Autodesk Fusion 360 part; units mm, degrees
sketch "Sketch1" plane through (0, 0, 0) normal (0, 0, 1) x (1, 0, 0)
  line L0 (0, 0) -> (23, 0)
  line L1 (23, 0) -> (23, 19)
  line L2 (23, 19) -> (0, 19)
  line L3 (0, 19) -> (0, 0)
  line L4 (0, 0) -> (23, 19) construction
  line L5 (14, -5.5) -> (9, -5.5) construction
  line L6 (9, -5.5) -> (9, 24.5)
  line L7 (9, 24.5) -> (14, 24.5) construction
  line L8 (14, 24.5) -> (14, -5.5)
  line L9 (14, -5.5) -> (9, 24.5) construction
  line L10 (9, -5.5) -> (14, 24.5) construction
  line L11 (-3, 22) -> (-3, -3)
  line L12 (-3, -3) -> (26, -3)
  line L13 (26, -3) -> (26, 22)
  line L14 (26, 22) -> (-3, 22)
  point P0 (11.5, 9.5)
  dimension "d1" = 23
  dimension "d2" = 19
  dimension "d5" = 5
  dimension "d6" = 3
  dimension "d11" = 30
extrude "Extrude4" add sketch "Sketch1" along normal blind 50 contours L0 L2 L3 L6 L11 L12 L14 | L0 L1 L2 L8 L12 L13 L14 makes body 1 at (-3, 13.6667, 16.6667) makes body 2 at (26, 5.3333, 16.6667)
sketch "Sketch2" plane through (0, 0, 50) normal (0, 0, 1) x (-1, 0, 0)
  line L0 (-14, 0) -> (-14, 3)
  line L1 (-14, 3) -> (-26, 3)
  line L2 (-26, 3) -> (-26, -22)
  line L3 (-26, -22) -> (-14, -22)
  line L4 (-14, -22) -> (-14, -19)
  line L5 (-14, -19) -> (-23, -19)
  line L6 (-23, -19) -> (-23, 0)
  line L7 (-23, 0) -> (-14, 0)
  line L8 (0.208, -22.1542) -> (-23, -22.1542)
  line L9 (-23, -22.1542) -> (-23, -19)
  line L10 (-23, -19) -> (0.208, -19)
  line L11 (0.208, -19) -> (0.208, -22.1542)
  line L12 (0, 0) -> (-23, 0)
  line L13 (-23, 0) -> (-23, 3)
  line L14 (-23, 3) -> (0, 3)
  line L15 (0, 3) -> (0, 0)
extrude "Extrude5" add sketch "Sketch2" against normal blind 10 contours L0 L1 L7 L12 L13 L14 | L0 L12 L14 L15 | L3 L4 L5 L9 L10 | L3 L4 L8 L9 L10 L11 bodies 1 2
copy_body "CopyPasteBodies1" bodies 1 makes body 3
move_body "Move1" bodies 3 to x (1, 0, 0) y (0, 1, 0) z (0, 0, 1) at (0, 30, 0)
move_body "Move2" bodies 3 to x (1, 0, 0) y (0, 1, 0) z (0, 0, 1) at (0, -5, 0)
sketch "Sketch3" plane through (0, 0, 50) normal (0, 0, 1) x (-1, 0, 0)
  line L0 (0, -44) -> (-23, -44)
  line L1 (-23, -44) -> (-23, -25)
  line L2 (-23, -25) -> (0, -25)
  line L3 (0, -25) -> (0, -44)
  line L4 (-23, -47) -> (-23, -47.1542)
  line L5 (-23, -47.1542) -> (0.208, -47.1542)
  line L6 (0.208, -47.1542) -> (0.208, -47)
  line L7 (0.208, -47) -> (3, -47)
  line L8 (3, -47) -> (3, -22)
  line L9 (3, -22) -> (-26, -22)
  line L10 (-26, -22) -> (-26, -47)
  line L11 (-26, -47) -> (-23, -47)
  line L12 (0, 0) -> (-23, -44) construction
  line L13 (26, 7) -> (-49, 7)
  line L14 (-49, 7) -> (-49, -51)
  line L15 (-49, -51) -> (26, -51)
  line L16 (26, -51) -> (26, 7)
  line L17 (26, 7) -> (-49, -51) construction
  line L18 (-49, 7) -> (26, -51) construction
  line L19 (-49, -51) -> (-43, -51) construction
  line L20 (-43, -51) -> (-43, 7)
  line L21 (13.676, 7) -> (-5, 7)
  line L22 (-5, 7) -> (-5, -1)
  line L23 (-5, -1) -> (13.676, -1)
  line L24 (13.676, -1) -> (13.676, 7)
  line L25 (10.3139, -51) -> (-3.2871, -51)
  line L26 (-3.2871, -51) -> (-3.2871, -42.2509)
  line L27 (-3.2871, -42.2509) -> (10.3139, -42.2509)
  line L28 (10.3139, -42.2509) -> (10.3139, -51)
  point P0 (-11.5, -22)
  point P1 (3, -46.6655)
  point P2 (4.6174, 2.0386)
  dimension "d16" = 75
  dimension "d17" = 58
  dimension "d22" = 6
  dimension "d23" = 8
extrude "Extrude6" add sketch "Sketch3" along normal blind 1 and the other way blind 1 bodies 1 3
extrude "Extrude7" add sketch "Sketch3" along normal blind 25 contours L0 L3 L5 L6 L7 L8 L26 L27 | L0 L3 L26 L27 | L5 L6 L7 L8 L15 L25 L26 L27 L28 | L13 L14 L15 L20 | L13 L21 L22 L23 L24 bodies 1
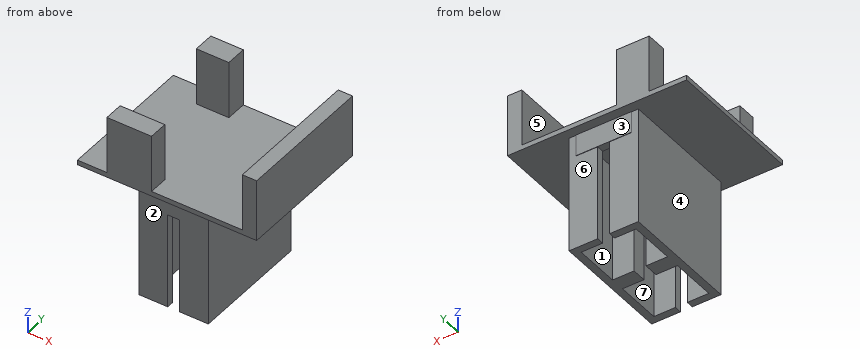
Part model, mm, in its own coordinate system. Face numbers are marked on the shaded views. A direction names the side the tool comes from. Round coordinates to 2 decimals unless told otherwise and drop trailing zeros. Order: outer loops, then holes, each group sorted by start corner. A loop starts at its lowest first (then second) coordinate and runs counter-clockwise, first axis right, second up. Notation, with made-up numbers: (87.5, 46) -> (107.5, 46) arc R31 ccw to (107.5, 77) -> close; hole circle Ø6 at (77.25, 20.25). An arc over 180 degrees is marked (long way). Put each result on its own line as item: value.
Q1. Pull direction X, two halves, no side cores. Call the marked faces 4, 5, 6 and 7: pulls with the +X half, pulls with the -X half, needs draft (parallel to the pull), parting line crosses it, or undercut.
From the geometry:
face 4: pulls with the -X half
face 5: undercut
face 6: needs draft
face 7: undercut
Q2. Band-saw the part on B-B (z = 17). Give the cut face in (x, y), and give its area (3 significant figures).
From the geometry:
outline: (-3, -3) -> (9, -3) -> (9, 0) -> (0, 0) -> (0, 19) -> (9, 19) -> (9, 25) -> (0, 25) -> (0, 44) -> (9, 44) -> (9, 47) -> (-3, 47) -> close; (14, -3) -> (26, -3) -> (26, 47) -> (14, 47) -> (14, 44) -> (23, 44) -> (23, 25) -> (14, 25) -> (14, 19) -> (23, 19) -> (23, 0) -> (14, 0) -> close
area: 516 mm2
Q3. Band-saw the part on A-A (z = 70). Give the cut face in (x, y), and give its area (3 significant figures).
From the geometry:
outline: (-13.68, -7) -> (5, -7) -> (5, 1) -> (-13.68, 1) -> close; (-10.31, 42.25) -> (3.29, 42.25) -> (3.29, 51) -> (-10.31, 51) -> close; (43, -7) -> (49, -7) -> (49, 51) -> (43, 51) -> close
area: 616 mm2
Q4. Band-saw the part on C-C (y = 23). Give the cut face in (x, z), and give its area (4 significant figures).
From the geometry:
outline: (-26, 49) -> (-3, 49) -> (-3, 0) -> (9, 0) -> (9, 40) -> (14, 40) -> (14, 0) -> (26, 0) -> (26, 49) -> (49, 49) -> (49, 75) -> (43, 75) -> (43, 51) -> (-26, 51) -> close
area: 1,515 mm2
Q5. Wall check: line 1 (Y direction, x = 5, z = 48.5); line 2 (X direction, y = 30, z = 27.5); line 3 (Z direction, x = -10.5, y = 38). Give the ranges that are in metal, low to high. Write a range as [from, to].
From the geometry:
line 1: y = [-3, 0], [19, 25], [44, 47.15]
line 2: x = [-3, 0], [23, 26]
line 3: z = [49, 51]
Q6. Pin check, flat tips, straight feed: pin 1 Ø7 at (x, z) = (9, 24) entering from +Y; pin 2 Ø2 at (x, y) = (13.5, 5) entering from +Z; pin 3 Ø0.9 at (y, z) = (-1, 10.5) entering from -X. Stop position of each tip, or through.
From the geometry:
pin 1: stops at y = 47
pin 2: stops at z = 51
pin 3: stops at x = -3
Q7. Tool access for the marked faces 1, 2 and 3: list every direction of +Z, -Z, +X, -X, +Y, -Y with a clear straight run to the whole face (end or side of a thin tool).
From the geometry:
face 1: -Z
face 2: -Z, +X, -X, -Y
face 3: -Z, +X, -X, +Y
Q8. Band-saw the part on D-D (x = 6). Give the cut face in (y, z).
From the geometry:
outline: (-7, 49) -> (-3, 49) -> (-3, 0) -> (0, 0) -> (0, 49) -> (19, 49) -> (19, 0) -> (25, 0) -> (25, 49) -> (44, 49) -> (44, 0) -> (47, 0) -> (47, 40) -> (47.15, 40) -> (47.15, 49) -> (51, 49) -> (51, 51) -> (-7, 51) -> close
